from build123d import *

# Parameters (mm, degrees)
F0_W     = 70.852228
F0_H     = 70.129245
F1_DEPTH = 25.4
F2_W     = 67.719309
F2_H     = 100.253496
F3_DEPTH = 36.322
F4_W     = 67.960299
F4_H     = 100.253489
F5_DEPTH = 30.734


with BuildPart() as f1:
    # F0 (on Front) → F1 (new body)
    with BuildSketch(Plane.XZ):
        with Locations((0.722982, -10.00125)):
            Rectangle(F0_W, F0_H)
    extrude(amount=F1_DEPTH)

    # F2 (on Right) → F3 (join)
    with BuildSketch(Plane.YZ):
        with Locations((-10.965226, -8.675782)):
            Rectangle(F2_W, F2_H)
    extrude(amount=F3_DEPTH)

    # F4 (on face) → F5 (join)
    with BuildSketch(Plane(origin=(-34.703132, 0, 0), x_dir=(0, -1, 0), z_dir=(-1, 0, 0))):
        with Locations((11.085722, -8.434789)):
            Rectangle(F4_W, F4_H)
    extrude(amount=F5_DEPTH)


solid = f1.part
Input: part model. Units: mm. Frame: model coordinates. A direction names the side the tool comes from. Round coordinates to 2 decimals unless told otherwise and drop trailing zeros. Order: outer loops, then holes, each group sorted by start corner. A loop starts at its lowest first (then second) coordinate and runs counter-clockwise, first axis right, second up. Notation, with made-up numbers: (61, 77.5) - (117, 77.5) arc R18 cw to (117, 109.5) - close; hole circle Ø5 at (-16.5, -29). An arc over 180 degrees is marked (long way). Use a Markdown table: item, result.
1. Section A-A on z = 28. Return the cut outline in (x, y), then the cut area to 3 significant figures.
Evaluation:
| item | result |
|---|---|
| outline | (-65.44, -45.07) - (-34.7, -45.07) - (-34.7, 22.89) - (-65.44, 22.89) - close; (0, -44.82) - (36.32, -44.82) - (36.32, 22.89) - (0, 22.89) - close |
| area | 4,550 mm^2 |
2. Section B-B on y = 15. Return the cut outline in (x, z).
Evaluation:
| item | result |
|---|---|
| outline | (-65.44, -58.56) - (-34.7, -58.56) - (-34.7, 41.69) - (-65.44, 41.69) - close; (0, -58.8) - (36.32, -58.8) - (36.32, 41.45) - (0, 41.45) - close |
3. First-contact query: pin 1 (4 mm diameter, centred on x = -22.5, z = -11.5, fed in from +Y); pin 2 (20.5 mm diameter, centred on x = -12.5, y = -15, fed in from -Z); pin 3 (2 mm diameter, centred on x = -4.5, y = -15, fed in from +Z). Flat tips, straight axial feed; report the tip coordinate or a pass-through.
Evaluation:
| item | result |
|---|---|
| pin 1 | y = 0 |
| pin 2 | z = -45.07 |
| pin 3 | z = 25.06 |
4. Access query for faces 1 (the face through (18, -11, 41.451)), 2 (the face through (-18, -25.4, -10)), 3 (the face through (-18, -13, -45.066)). Directions: +Z, -Z, +X, -X, +Y, -Y. A direction counts if a zero-diameter tool reaches every point of the face in a straight line with its end or side. Return the directions, or none.
Evaluation:
| item | result |
|---|---|
| face 1 | +Z, +X, +Y, -Y |
| face 2 | +Z, -Z, -Y |
| face 3 | -Z, +Y, -Y |
5. Section C-C on y = -6. Return the cut outline in (x, z), then the cut area to 3 significant figures.
Evaluation:
| item | result |
|---|---|
| outline | (-65.44, -58.56) - (-34.7, -58.56) - (-34.7, -45.07) - (0, -45.07) - (0, -58.8) - (36.32, -58.8) - (36.32, 41.45) - (0, 41.45) - (0, 25.06) - (-34.7, 25.06) - (-34.7, 41.69) - (-65.44, 41.69) - close |
| area | 9,160 mm^2 |
6. Section D-D on z = -43.5. Return the cut outline in (x, y), then the cut area to 3 significant figures.
Evaluation:
| item | result |
|---|---|
| outline | (-65.44, -45.07) - (-34.7, -45.07) - (-34.7, -25.4) - (0, -25.4) - (0, -44.82) - (36.32, -44.82) - (36.32, 22.89) - (0, 22.89) - (0, 0) - (-34.7, 0) - (-34.7, 22.89) - (-65.44, 22.89) - close |
| area | 5,430 mm^2 |
7. Mould query, pull axis X, two halves, no side actions, for faces 4 (the face through (-18, 0, -10)), 5 (the face through (-65.437, -11, -8)), 6 (the face through (36.322, -11, -8)). Classes: +X half, -X half, draft (parallel to the pull), parting line (faces both ways), or undercut.
Evaluation:
| item | result |
|---|---|
| face 4 | undercut |
| face 5 | -X half |
| face 6 | +X half |
8. Material intervals for probe 1 along X at (y, z) = (15.5, 15); probe 2 along Y at (x, z) = (5.5, 34.5); probe 3 along Y at (x, z) = (-34.5, 5.5), sorted ascending.
Evaluation:
| item | result |
|---|---|
| probe 1 | -65.44 to -34.7, 0 to 36.32 |
| probe 2 | -44.82 to 22.89 |
| probe 3 | -25.4 to 0 |
